Could you check a few things on this model? Use its own coordinates, in mm. A direction names the side the tool comes from. Coordinates: 2 decimals unless noted, no trailing zeros. Order: outer loops, then holes, each group sorted by start corner. A loop starts at its lowest first (then second) coordinate and runs counter-clockwise, first axis right, second up. Notation, with made-up numbers: (78, 61.25) -> (137, 61.25) arc R17 ccw to (137, 71.25) -> close; hole circle Ø11 at (-12, 21.25). An arc over 180 degrees is marked (long way). Put each result on its own line as item: value. Start each with the question number.
Q1. For faces 5 (the face through (-26, -1031, -10)), 6 (the face through (-104.088, -1032, -80)), 7 (the face through (-115.338, -1031, -635)), 8 (the face through (-170, -1031, -10)), which set-ups out of +Z, -Z, +X, -X, +Y, -Y let a thin tool reach every point of the face, with its end or its side?
Q2. If we section it at A-A (y = -1030.5): Count the separate pieces of the cut face and the enclosed holes in it, and give its area (3 significant figures).
Q3. If we section it at B-B (x = -21.5): Please give me the cut outline in (y, z).
Q4. We'd pull the mould along Z, two halves only. Please class faces 1 (the face through (-64, -1031, 0)), 2 (the face through (-108.088, -1032, -368)), 3 (the face through (-170, -1031, -630)), 4 (the face through (-108.088, -1032, -80)): +Z half, -Z half, draft (parallel to the pull), parting line (faces both ways), or undercut.
Q5. Will these pins go through, and if not, where does the flat tip stop? pin 1 (5 mm diameter, centred on y = -1031.5, z = -5, fed in from +X); pin 2 (3 mm diameter, centred on y = -1035, z = -633.5, fed in from -X); pin 3 (2.5 mm diameter, centred on x = -97.84, z = -192, fed in from -Y).
Q6. Please list where these lines run through material, in increasing order: line 1 along Z through (x, y) = (-63, -1026.75); line 2 along Z through (x, y) = (-106.5, -1031.5); line 3 along X through (y, z) = (-1026.25, -635).
from build123d import *

# Parameters (mm, degrees)
SKETCH1_W                    = 184
SKETCH1_H                    = 18
BOSS_EXTRUDE1_DEPTH          = 658
CAVITY1_START                = -10
CAVITY1_OUTLINE_W            = 35
CAVITY1_OUTLINE_H            = 18
CAVITY1_OUTLINE_R            = 1.5
CAVITY1_OUTLINE_W_2          = 40.7
CAVITY1_DEPTH                = 10
CAVITY2_START                = -640
CAVITY2_OUTLINE_W            = 35
CAVITY2_OUTLINE_H            = 18
CAVITY2_OUTLINE_R            = 1.5
CAVITY2_OUTLINE_W_2          = 40.7
CAVITY2_DEPTH                = 10
SKETCH2_W                    = 184
SKETCH2_H                    = 18
CUT_EXTRUDE1_DEPTH           = 20
F_3_0_3_DIAMETER_HOLE1_D     = 3
F_3_0_3_DIAMETER_HOLE1_DEPTH = 25
F_3_0_3_DIAMETER_HOLE1_TIP   = 0.901290929
SKETCH5_W                    = 15.438081993
SKETCH5_H                    = 17.38610898
SKETCH5_W_2                  = 12.462066187
SKETCH5_W_3                  = 22.69212052
SKETCH5_W_4                  = 24.151046806
SKETCH5_H_2                  = 18.747641983
SKETCH5_W_5                  = 17.028403492
SKETCH5_H_3                  = 21.404849388
SKETCH5_W_6                  = 27.020251182
CUT_EXTRUDE2_DEPTH           = 20
F_3_0_3_DIAMETER_HOLE2_D     = 3
F_3_0_3_DIAMETER_HOLE2_DEPTH = 5
F_3_0_3_DIAMETER_HOLE2_TIP   = 0.901290929
CUT_EXTRUDE3_DEPTH           = 16


# Read off the part's stored shape, not the designer's step: Cavity1, Cavity2
with BuildPart() as part:
    # Sketch1 → Boss-Extrude1 (new body)
    with BuildSketch(Plane.XY):
        with Locations((-97.838367622, -1030.94)):
            Rectangle(SKETCH1_W, SKETCH1_H)
    extrude(amount=-BOSS_EXTRUDE1_DEPTH)

    # Cavity1 outline → Cavity1 (cut)
    # profile 1 of 3: a face of its own
    with BuildSketch(Plane.XY.offset(CAVITY1_START)):
        with Locations((-97.838367622, -1030.94)):
            Rectangle(CAVITY1_OUTLINE_W, CAVITY1_OUTLINE_H)
        with Locations((-97.838367622, -1030.94)):
            Circle(CAVITY1_OUTLINE_R, mode=Mode.SUBTRACT)
    # profile 2 of 3: a face of its own
    with BuildSketch(Plane.XY.offset(CAVITY1_START)):
        with Locations((-169.488367622, -1030.94)):
            Rectangle(CAVITY1_OUTLINE_W_2, CAVITY1_OUTLINE_H)
        with Locations((-169.488367622, -1030.94)):
            Circle(CAVITY1_OUTLINE_R, mode=Mode.SUBTRACT)
    # profile 3 of 3: a face of its own
    with BuildSketch(Plane.XY.offset(CAVITY1_START)):
        with Locations((-26.188367622, -1030.94)):
            Rectangle(CAVITY1_OUTLINE_W_2, CAVITY1_OUTLINE_H)
        with Locations((-26.188367622, -1030.94)):
            Circle(CAVITY1_OUTLINE_R, mode=Mode.SUBTRACT)
    extrude(amount=CAVITY1_DEPTH, mode=Mode.SUBTRACT)

    # Cavity2 outline → Cavity2 (cut)
    # profile 1 of 3: a face of its own
    with BuildSketch(Plane.XY.offset(CAVITY2_START)):
        with Locations((-97.838367622, -1030.94)):
            Rectangle(CAVITY2_OUTLINE_W, CAVITY2_OUTLINE_H)
        with Locations((-97.838367622, -1030.94)):
            Circle(CAVITY2_OUTLINE_R, mode=Mode.SUBTRACT)
    # profile 2 of 3: a face of its own
    with BuildSketch(Plane.XY.offset(CAVITY2_START)):
        with Locations((-169.488367622, -1030.94)):
            Rectangle(CAVITY2_OUTLINE_W_2, CAVITY2_OUTLINE_H)
        with Locations((-169.488367622, -1030.94)):
            Circle(CAVITY2_OUTLINE_R, mode=Mode.SUBTRACT)
    # profile 3 of 3: a face of its own
    with BuildSketch(Plane.XY.offset(CAVITY2_START)):
        with Locations((-26.188367622, -1030.94)):
            Rectangle(CAVITY2_OUTLINE_W_2, CAVITY2_OUTLINE_H)
        with Locations((-26.188367622, -1030.94)):
            Circle(CAVITY2_OUTLINE_R, mode=Mode.SUBTRACT)
    extrude(amount=CAVITY2_DEPTH, mode=Mode.SUBTRACT)

    # Sketch2 → Cut-Extrude1 (cut)
    with BuildSketch(Plane.XZ.offset(1039.94)):
        with Locations((-97.838367622, -649)):
            Rectangle(SKETCH2_W, SKETCH2_H)
    extrude(amount=-CUT_EXTRUDE1_DEPTH, mode=Mode.SUBTRACT)

    # Ø3.0 (3) Diameter Hole1
    with Locations(Plane(origin=(0, -1039.94, 0), x_dir=(-1, 0, 0), z_dir=(0, -1, 0))):
        with Locations((132.238367622, 5), (63.438367622, 5), (63.438367622, 635), (132.238367622, 635)):
            Hole(F_3_0_3_DIAMETER_HOLE1_D / 2, depth=F_3_0_3_DIAMETER_HOLE1_DEPTH)
            with Locations((0, 0, -(F_3_0_3_DIAMETER_HOLE1_DEPTH + F_3_0_3_DIAMETER_HOLE1_TIP / 2))):  # 118° drill point
                Cone(0, F_3_0_3_DIAMETER_HOLE1_D / 2, F_3_0_3_DIAMETER_HOLE1_TIP, mode=Mode.SUBTRACT)

    # Sketch5 → Cut-Extrude2 (cut)
    with BuildSketch(Plane.XZ.offset(1039.94)):
        with Locations((-168.439296688, -638.69305449)):
            Rectangle(SKETCH5_W, SKETCH5_H)
        with Locations((-97.014917346, -638.69305449)):
            Rectangle(SKETCH5_W_2, SKETCH5_H)
        with Locations((-26.055540475, -638.69305449)):
            Rectangle(SKETCH5_W_3, SKETCH5_H)
        with Locations((-172.795779094, -0.626179008)):
            Rectangle(SKETCH5_W_4, SKETCH5_H_2)
        with Locations((-99.298085999, 0.702424694)):
            Rectangle(SKETCH5_W_5, SKETCH5_H_3)
        with Locations((-23.891475144, 0.702424694)):
            Rectangle(SKETCH5_W_6, SKETCH5_H_3)
    extrude(amount=-CUT_EXTRUDE2_DEPTH, mode=Mode.SUBTRACT)

    # Ø3.0 (3) Diameter Hole2
    with Locations(Plane(origin=(0, -1039.94, 0), x_dir=(-1, 0, 0), z_dir=(0, -1, 0))):
        with Locations((97.838367622, 64), (97.838367622, 384), (97.838367622, 576), (97.838367622, 192), (97.838367622, 15.63)):
            Hole(F_3_0_3_DIAMETER_HOLE2_D / 2, depth=F_3_0_3_DIAMETER_HOLE2_DEPTH)
            with Locations((0, 0, -(F_3_0_3_DIAMETER_HOLE2_DEPTH + F_3_0_3_DIAMETER_HOLE2_TIP / 2))):  # 118° drill point
                Cone(0, F_3_0_3_DIAMETER_HOLE2_D / 2, F_3_0_3_DIAMETER_HOLE2_TIP, mode=Mode.SUBTRACT)

    # Sketch8 → Cut-Extrude3 (cut)
    with BuildSketch(Plane.XZ.offset(1039.94)):
        with BuildLine():
            Line((-108.088367622, -85.802173793), (-108.088367622, -74.197826207))
            ThreePointArc((-108.088367622, -74.197826207), (-106.088367622, -72.197826207), (-104.088367622, -74.197826207))
            Line((-104.088367622, -74.197826207), (-104.088367622, -85.802173793))
            ThreePointArc((-104.088367622, -85.802173793), (-106.088367622, -87.802173793), (-108.088367622, -85.802173793))
        make_face()
        with BuildLine():
            Line((-108.088367622, -373.121722836), (-108.088367622, -362.878277164))
            ThreePointArc((-108.088367622, -362.878277164), (-106.088367622, -360.878277164), (-104.088367622, -362.878277164))
            Line((-104.088367622, -362.878277164), (-104.088367622, -373.121722836))
            ThreePointArc((-104.088367622, -373.121722836), (-106.088367622, -375.121722836), (-108.088367622, -373.121722836))
        make_face()
        with BuildLine():
            Line((-108.088367622, -565.121722836), (-108.088367622, -554.878277164))
            ThreePointArc((-108.088367622, -554.878277164), (-106.088367622, -552.878277164), (-104.088367622, -554.878277164))
            Line((-104.088367622, -554.878277164), (-104.088367622, -565.121722836))
            ThreePointArc((-104.088367622, -565.121722836), (-106.088367622, -567.121722836), (-108.088367622, -565.121722836))
        make_face()
    extrude(amount=-CUT_EXTRUDE3_DEPTH, mode=Mode.SUBTRACT)


solid = part.part
The answers:
1. face 5: +Z, +X, +Y, -Y
1. face 6: -Y
1. face 7: -Z, +Y, -Y
1. face 8: +Z, -X, +Y, -Y
2. separate pieces: 1
2. enclosed holes: 7
2. area: 115,000 mm^2
3. outline: (-1039.94, -630) -> (-1021.94, -630) -> (-1021.94, -10) -> (-1039.94, -10) -> close
4. face 1: +Z half
4. face 2: undercut
4. face 3: -Z half
4. face 4: undercut
5. pin 1: x = -46.54
5. pin 2: x = -149.14
5. pin 3: y = -1034.79
6. line 1: -640 to -636.43, -633.57 to -6.43, -3.57 to 0
6. line 2: -630 to -567.08, -552.92 to -375.08, -360.92 to -87.76, -72.24 to -10
6. line 3: -149.14 to -133.74, -130.74 to -115.34, -80.34 to -64.94, -61.94 to -46.54
